Check sheet for the drawn part. Datum: minimum x, y, z corner. Units: mm. A direction names the side the tool comes from. Give positions to 0.01 mm unless a question says otherwise; leave off trailing zeros. Write each loop counter-clockwise with the first axis right and the second up, starting at its lowest first coordinate (ties: lowest second). Pieces come first, ordered by that corner, then holes. Notation, with made-up numbers: (84.25, 31) -> (89.25, 31) arc R24 ccw to (89.25, 42) -> close; hole circle Ø1 at (38.5, -34.5). An arc over 180 degrees is marked (long way). Answer as CSV lines item,"result". Start each with the question number.
1) Gauge pin test, flat ends, axial feed: pin 1 Ø13 at (x, z) = (25, 25) entering from -Y; pin 2 Ø3 at (x, y) = (22, 2.5) entering from +Z; pin 3 Ø6.5 at (x, z) = (29.5, 29) entering from +Y. Record the tip position at first contact, or that the pin passes through.
2) Sectioned sample at B-B on x = 25. Record the cut outline in (y, z), and give its area (3 significant figures).
3) Material ranges on L1, parallel to X at y = 2.05, z = 25; L2, parallel to X at y = 6, z = 25; L3, parallel to Y at x = 25.5, z = 19.5, recorded low to high.
4) Sectioned sample at A-A on z = 25. Record the cut outline in (x, y), and give its area (3 significant figures).
5) Sectioned sample at D-D on x = 31. Record the cut outline in (y, z).
6) Sectioned sample at C-C on y = 3.75. Record the cut outline in (x, z).
7) Mould release check, pull along X, two halves, no side actions. Record for the marked faces 3, 4, 5 and 6: released by +X, released by -X, zero draft, split by the parting line, or undercut.
8) Tool access check on the marked faces 1 and 2. Record the directions out of +Z, -Z, +X, -X, +Y, -Y that give a thin tool (end or side, any length) a straight path to the whole face; none if there is none.
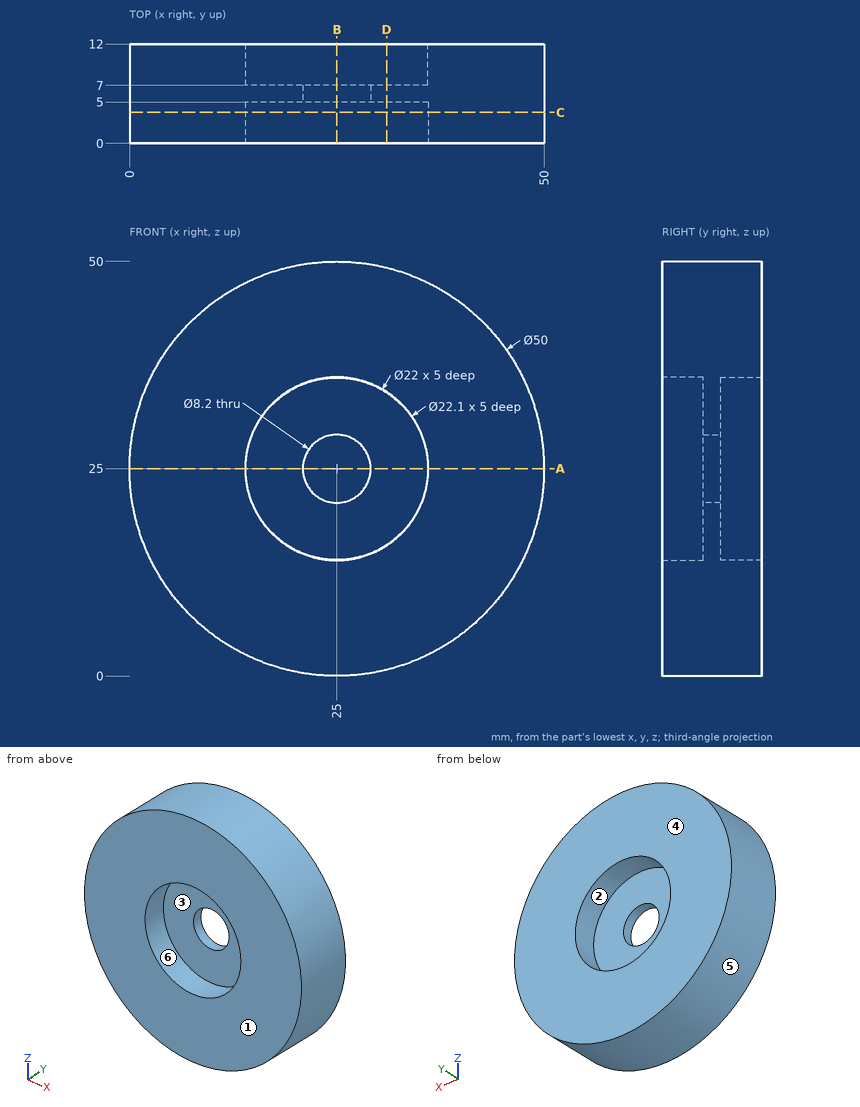
Ans:
1,pin 1,"stops at y = 5"
1,pin 2,"stops at z = 49.95"
1,pin 3,"stops at y = 7"
2,outline,"(0, 0) -> (12, 0) -> (12, 14) -> (7, 14) -> (7, 20.9) -> (5, 20.9) -> (5, 13.95) -> (0, 13.95) -> close; (0, 36.05) -> (5, 36.05) -> (5, 29.1) -> (7, 29.1) -> (7, 36) -> (12, 36) -> (12, 50) -> (0, 50) -> close"
2,area,"363 mm²"
3,L1,"x = 0 to 13.95, 36.05 to 50"
3,L2,"x = 0 to 20.9, 29.1 to 50"
3,L3,"y = 5 to 7"
4,outline,"(0, 0) -> (13.95, 0) -> (13.95, 5) -> (20.9, 5) -> (20.9, 7) -> (14, 7) -> (14, 12) -> (0, 12) -> close; (29.1, 5) -> (36.05, 5) -> (36.05, 0) -> (50, 0) -> (50, 12) -> (36, 12) -> (36, 7) -> (29.1, 7) -> close"
4,area,"363 mm²"
5,outline,"(0, 0.73) -> (12, 0.73) -> (12, 15.78) -> (7, 15.78) -> (7, 34.22) -> (12, 34.22) -> (12, 49.27) -> (0, 49.27) -> (0, 34.28) -> (5, 34.28) -> (5, 15.72) -> (0, 15.72) -> close"
6,outline,"circle Ø50 at (25, 25); hole circle Ø22.1 at (25, 25)"
7,face 3,"undercut"
7,face 4,"zero draft"
7,face 5,"split by the parting line"
7,face 6,"undercut"
8,face 1,"+Z, -Z, +X, -X, -Y"
8,face 2,"+Y"
